Geometry check sheet. Reference: the model listing, model coordinates, mm. A direction names the side the tool comes from. Give positions to 0.01 mm unless a question says otherwise; leave off trailing zeros. Order: outer loops, then holes, each group sorted by start corner. A loop starts at its lowest first (then second) coordinate and runs counter-clockwise, first axis right, second up. Notation, with made-up numbers: M 43,7.25 L 62,7.25 A22 cw 62,34.25 Z; hole C 13.5,37.25 d9. An arc over 180 degrees is marked long. One line per question, with ' | ' between items. Start each with the question number.
from build123d import *

# Parameters (mm, degrees)
SKETCH1_W                = 7
SKETCH1_H                = 24
BOSS_EXTRUDE1_DEPTH      = 2.5
FILLET1_R                = 1
SKETCH2_R                = 7.5
BOSS_EXTRUDE2_DEPTH      = 0.5
BOSS_EXTRUDE2_DEPTH_BACK = 2.5
SKETCH3_R                = 1.05
CUT_EXTRUDE1_DEPTH       = 22.5
SKETCH5_R                = 1.561205439
BOSS_EXTRUDE3_DEPTH      = 0.5
SKETCH6_R                = 4
BOSS_EXTRUDE4_DEPTH      = 3.7


with BuildPart() as part:
    # Sketch1 → Boss-Extrude1 (new body)
    with BuildSketch(Plane(origin=(0, 0, 0), x_dir=(1, 0, 0), z_dir=(0, 1, 0))):
        Rectangle(SKETCH1_W, SKETCH1_H)
    extrude(amount=BOSS_EXTRUDE1_DEPTH)

    # Fillet1
    fillet1_edges = [part.edges().sort_by_distance(p)[0] for p in [
        (3.5, 1.25, 12),
        (-3.5, 1.25, 12),
        (-3.5, 1.25, -12),
        (3.5, 1.25, -12),
    ]]
    fillet(fillet1_edges, radius=FILLET1_R)

    # Sketch2 → Boss-Extrude2 (add, two sides)
    with BuildSketch(Plane(origin=(0, 2.5, 0), x_dir=(1, 0, 0), z_dir=(0, 1, 0))) as boss_extrude2_sk:
        Circle(SKETCH2_R)
    extrude(amount=BOSS_EXTRUDE2_DEPTH)
    extrude(boss_extrude2_sk.sketch, amount=-BOSS_EXTRUDE2_DEPTH_BACK)

    # Sketch3 → Cut-Extrude1 (cut)
    with BuildSketch(Plane(origin=(0, 2.5, 0), x_dir=(1, 0, 0), z_dir=(0, 1, 0))):
        with Locations((0, 9.5)):
            Circle(SKETCH3_R)
        with Locations((0, -9.5)):
            Circle(SKETCH3_R)
    extrude(amount=-CUT_EXTRUDE1_DEPTH, mode=Mode.SUBTRACT)

    # Sketch5 → Boss-Extrude3 (add)
    with BuildSketch(Plane(origin=(0, 3, 0), x_dir=(1, 0, 0), z_dir=(0, 1, 0))):
        Circle(SKETCH5_R)
    extrude(amount=BOSS_EXTRUDE3_DEPTH)

    # Sketch6 → Boss-Extrude4 (add)
    with BuildSketch(Plane(origin=(0, 3.5, 0), x_dir=(1, 0, 0), z_dir=(0, 1, 0))):
        Circle(SKETCH6_R)
    extrude(amount=BOSS_EXTRUDE4_DEPTH)


solid = part.part
Item 1: Cross-section at B-B, the plane x = 0. Record the cut outline in (y, z), plus the area to 3 significant figures.
Item 2: Set-up check for faces 4 (the flat face through (-3.5, 1, 9)), 5 (the cylindrical face through (3.199, 1.268, 11.715)), 6 (the cylindrical face through (0.56, 1.27, -10.39)), 7 (the cylindrical face through (-0.867, 5.324, 3.905)), 8 (the flat face through (2, 3.5, 0)): record each of +Z, -Z, +X, -X, +Y, -Y from which the full face is reachable in a straight line by a thin tool's end or side.
Item 3: Cross-section at D-D, the plane y = 4.25. Record the cut outline in (x, z), plus the area to 3 significant figures.
Item 4: Cross-section at C-C, the plane z = 0. Record the cut outline in (x, y), plus the area to 3 significant figures.
Item 5: Depth check by flat-ended pin: pin 1 (4.5 mm diameter, centred on x = -0.5, z = 9.5, fed in from +Y); pin 2 (2.5 mm diameter, centred on x = 0, z = 9.5, fed in from +Y); pin 3 (3 mm diameter, centred on y = 1, z = -8.5, fed in from -X); pin 4 (1.5 mm diameter, centred on x = 4.5, z = 7, fed in from +Y). Enter the tip coordinate at first touch or a pass-through.
Item 6: Cross-section at A-A, the plane z = 9.5. Record the cut outline in (x, y), plus the area to 4 significant figures.
Item 7: Mould release check, pull along Z, two halves, no side actions. Record for faces 1 (the cylindrical face through (-3.215, 1.268, -11.699)), 2 (the cylindrical face through (0.56, 1.27, 8.61)), 3 (the flat face through (0.7, 2.5, 10.5)): released by +Z, released by -Z, zero draft, split by the parting line, or undercut.
Item 8: Material ranges on line 1 along Z through (x, y) = (0, 1); line 2 along Z through (x, y) = (0.75, 2); line 3 along X through (y, z) = (1.35, -9.5), recorded low to high.
Outcome:
1) outline: M 0,-12 L 2.5,-12 L 2.5,-10.55 L 0,-10.55 Z; M 0,-8.45 L 2.5,-8.45 L 2.5,-7.5 L 3,-7.5 L 3,-1.56 L 3.5,-1.56 L 3.5,-4 L 7.2,-4 L 7.2,4 L 3.5,4 L 3.5,1.56 L 3,1.56 L 3,7.5 L 2.5,7.5 L 2.5,8.45 L 0,8.45 Z; M 0,10.55 L 2.5,10.55 L 2.5,12 L 0,12 Z | area: 88.2 mm²
2) face 4: +Z, -X, +Y, -Y | face 5: +Z, +X, +Y, -Y | face 6: +Y, -Y | face 7: +Y | face 8: none
3) outline: C 0,0 d8 | area: 50.3 mm²
4) outline: M -7.5,0 L 7.5,0 L 7.5,3 L 1.56,3 L 1.56,3.5 L 4,3.5 L 4,7.2 L -4,7.2 L -4,3.5 L -1.56,3.5 L -1.56,3 L -7.5,3 Z | area: 76.2 mm²
5) pin 1: stops at y = 3 | pin 2: stops at y = 2.5 | pin 3: stops at x = -3.5 | pin 4: passes through
6) outline: M -3.5,0 L -1.05,0 L -1.05,2.5 L -3.5,2.5 Z; M 1.05,0 L 3.5,0 L 3.5,2.5 L 1.05,2.5 Z | area: 12.25 mm²
7) face 1: released by -Z | face 2: undercut | face 3: zero draft
8) line 1: z = -12 to -10.55, -8.45 to 8.45, 10.55 to 12 | line 2: z = -12 to -10.23, -8.77 to 8.77, 10.23 to 12 | line 3: x = -3.5 to -1.05, 1.05 to 3.5
